```python
from build123d import *

# Parameters (mm, degrees)
SALIENTE_EXTRUIR1_DEPTH = 87
SALIENTE_EXTRUIR2_START = -1
CROQUIS2_R              = 4
SALIENTE_EXTRUIR2_DEPTH = 1


with BuildPart() as part:
    # Croquis1 → Saliente-Extruir1 (new body)
    with BuildSketch(Plane.XY):
        with BuildLine():
            Line((-5.675682168, 13.871979869), (-13.577452672, 13.871979869))
            Line((-13.577452672, 13.871979869), (-13.577452672, -1.128020131))
            Line((-13.577452672, -1.128020131), (-6.693069658, -1.128020131))
            ThreePointArc((-6.693069658, -1.128020131), (1.75257721, 5.833649414), (-5.675682168, 13.871979869))
        make_face()
        with BuildLine():
            Line((-12.077452672, 12.371979869), (-5.877452672, 12.371979869))
            ThreePointArc((-5.877452672, 12.371979869), (0.122547328, 6.371979869), (-5.877452672, 0.371979869))
            Line((-5.877452672, 0.371979869), (-12.077452672, 0.371979869))
            Line((-12.077452672, 0.371979869), (-12.077452672, 12.371979869))
        make_face(mode=Mode.SUBTRACT)
    extrude(amount=SALIENTE_EXTRUIR1_DEPTH)

    # Croquis2 → Saliente-Extruir2 (add)
    with BuildSketch(Plane.XY.offset(87).offset(SALIENTE_EXTRUIR2_START)):
        with BuildLine():
            Line((-13.577452672, 13.871979869), (-13.577452672, -1.128020131))
            Line((-13.577452672, -1.128020131), (-4.825831505, -1.128020131))
            ThreePointArc((-4.825831505, -1.128020131), (1.757780912, 6.769060566), (-5.675682168, 13.871979869))
            Line((-5.675682168, 13.871979869), (-13.577452672, 13.871979869))
        make_face()
        with Locations((-6.077452672, 6.371979869)):
            Circle(CROQUIS2_R, mode=Mode.SUBTRACT)
    extrude(amount=SALIENTE_EXTRUIR2_DEPTH)


solid = part.part
```
Design review of the part built by this model. Coordinates are the model's own, in mm. A direction names the side the tool comes from. Give positions to 0.01 mm unless a question says otherwise; leave off trailing zeros. Loops run counter-clockwise (first coordinate to the right, second up) from the corner with the lowest first, then second, coordinate; pieces in that order, holes last. Notation, with made-up numbers: (-4.5, -39) -> (20.5, -39) arc R13 cw to (20.5, -19) -> close; hole circle Ø4 at (36.25, -34). An arc over 180 degrees is marked (long way). Write each question's results on one line, items separated by ' | '.
Q1. Machinability: for faces 4 (the face through (-6.598, 10.338, 86.493)), 5 (the face through (-12.077, 6, 42)), which of the approach directions +Z, -Z, +X, -X, +Y, -Y give a long, thin tool a straight path to every point of the face, cutting with its end or side? Answer none if there is none.
Reply:
face 4: +Z, -Z | face 5: -Z
Q2. For pin 1 Ø5 at (x, z) = (-8.5, 55) entering from -Y; pin 2 Ø6 at (x, y) = (-7.5, 7) entering from -Z; pin 3 Ø3.5 at (x, z) = (-11.5, 31) entering from -Y, all flat-tipped, find the tip position at first contact; note any pin that passes through.
Reply:
pin 1: stops at y = -1.18 | pin 2: stops at z = 86 | pin 3: stops at y = -1.13
Q3. Take a section at C-C, the plane x = -4. Write out the cut boundary in (y, z).
Reply:
outline: (-0.98, 0) -> (0.67, 0) -> (0.67, 86) -> (2.95, 86) -> (2.95, 87) -> (-0.98, 87) -> close; (9.79, 86) -> (12.07, 86) -> (12.07, 0) -> (13.66, 0) -> (13.66, 87) -> (9.79, 87) -> close
Q4. Take a section at B-B, the plane z = 19.5. Write out the cut boundary in (x, y).
Reply:
outline: (-13.58, -1.13) -> (-6.69, -1.13) arc R7.53 ccw (long way) to (-5.68, 13.87) -> (-13.58, 13.87) -> close; hole (-12.08, 0.37) -> (-5.88, 0.37) arc R6 ccw to (-5.88, 12.37) -> (-12.08, 12.37) -> close
Q5. Take a section at A-A, the plane y = 3.75. Write out the cut boundary in (x, z), plus the area to 3 significant figures.
Reply:
outline: (-13.58, 0) -> (-12.08, 0) -> (-12.08, 86) -> (-9.1, 86) -> (-9.1, 87) -> (-13.58, 87) -> close; (-3.06, 86) -> (-0.48, 86) -> (-0.48, 0) -> (1.31, 0) -> (1.31, 87) -> (-3.06, 87) -> close | area: 292 mm²
Q6. Wall thickness on L1, parallel to Y at x = -8.75, z = 56; L2, parallel to Y at x = -6, z = 60.5; L3, parallel to X at y = 6, z = 4.5: over which ranges is each line inside the solid? List them lowest first.
Reply:
L1: y = -1.13 to 0.37, 12.37 to 13.87 | L2: y = -1.18 to 0.37, 12.37 to 13.87 | L3: x = -13.58 to -12.08, 0.11 to 1.76
Q7. The part is to be moulded in two halves that separate along Y. For faces 1 (the face through (-10, -1.128, 43)), 2 (the face through (0.12, 6.5, 42.4)), 3 (the face through (-13.577, 6, 43)), say which applies: +Y half, -Y half, draft (parallel to the pull), parting line (faces both ways), or undercut.
Reply:
face 1: -Y half | face 2: undercut | face 3: draft
